Read the model definition and answer for the solid it produces. Units are mm, in the model's axes. Face numbers are marked on the shaded views. A direction names the side the tool comes from. Coordinates: 2 decimals unless noted, no trailing zeros. Order: outer loops, then holes, each group sorted by start corner. A loop starts at its lowest first (then second) coordinate and runs counter-clockwise, first axis right, second up. Notation, with made-up numbers: M 81.5,30 L 136.5,30 A20 ccw 136.5,43 Z; hole C 25,84 d3. An arc over 180 degrees is marked long. Use a Markdown table: item, result. Add a question column.
1) Find section C-C on z = 24.5. Write down the section's boundary in (x, y) (3 decimals).
2) Find the intervals of material crossed by probe 1 along X at (y, z) = (6, 21) (3 decimals); probe 2 along X at (y, z) = (-16.5, 46) (3 decimals); probe 3 along Z at (x, y) = (-22, 2.5) (3 decimals), in increasing order. Write a range as [from, to].
3) Find section A-A on z = 39. Write down the section's boundary in (x, y) (3 decimals), plus the area to 3 significant figures.
4) The mould has two halves that part along X. Classify the marked faces 4, 5 and 6: released by +X, released by -X, zero draft, split by the parting line, or undercut.
5) Find section B-B on x = -10. Write down the section's boundary in (y, z) (3 decimals).
6) Each of these flat-tipped pins is pushed along its axis until it touches: pin 1 Ø3 at (x, y) = (-11.5, 2.5) entering from +Z (3 decimals); pin 2 Ø9.5 at (y, z) = (-18, 46.5) entering from +X (3 decimals); pin 3 Ø12 at (x, z) = (14, 50) entering from -Y (3 decimals); pin 4 Ø9.5 at (y, z) = (-17, 32.5) entering from -X (3 decimals). Where does it stop, or does it pass through?
7) For the marked faces 1, 2 and 3, determine the directions among +Z, -Z, +X, -X, +Y, -Y from which every point of the face is accessible in a straight line to the end or side of a thin tool.
8) Find section D-D on y = 2.5. Write down the section's boundary in (x, z) (3 decimals), plus the area to 3 significant figures.
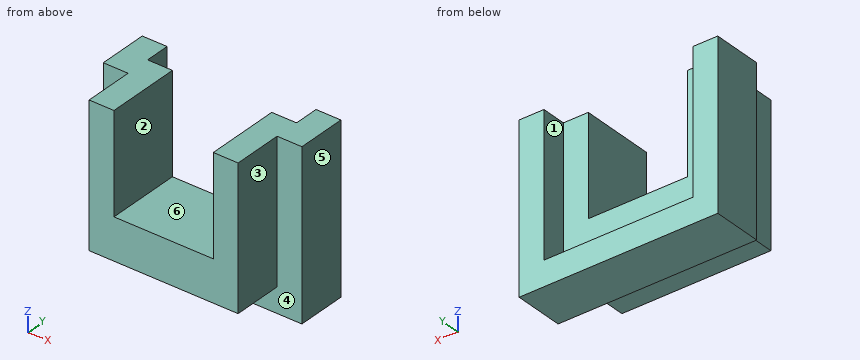
from build123d import *

# Parameters (mm, degrees)
BOSS_EXTRUDE1_DEPTH = 9.525
BOSS_EXTRUDE2_DEPTH = 28.575


with BuildPart() as part:
    # Sketch1 → Boss-Extrude1 (new, symmetric)
    with BuildSketch(Plane(origin=(0, 0, 0), x_dir=(1, 0, 0), z_dir=(0, 1, 0))):
        Polygon((38.1, 0), (-38.1, 0), (-38.1, -63.5), (-28.575, -63.5), (-28.575, -9.525), (28.575, -9.525), (28.575, -63.5), (38.1, -63.5), align=None)
    extrude(amount=BOSS_EXTRUDE1_DEPTH, both=True)

    # Sketch1<3> → Boss-Extrude2 (add)
    with BuildSketch(Plane(origin=(0, 0, 0), x_dir=(1, 0, 0), z_dir=(0, 1, 0))):
        Polygon((-28.575, -9.525), (-28.575, -63.5), (-19.05, -63.5), (-19.05, -25.4), (19.05, -25.4), (19.05, -63.5), (28.575, -63.5), (28.575, -9.525), align=None)
    extrude(amount=-BOSS_EXTRUDE2_DEPTH)


solid = part.part
Check result:
| question | item | result |
|---|---|---|
| 1 | outline | M -38.1,-9.525 L -28.575,-9.525 L -28.575,-28.575 L 28.575,-28.575 L 28.575,-9.525 L 38.1,-9.525 L 38.1,9.525 L 28.575,9.525 L 28.575,0 L -28.575,0 L -28.575,9.525 L -38.1,9.525 Z |
| 2 | probe 1 | x = [-38.1, -28.575], [28.575, 38.1] |
| 2 | probe 2 | x = [-28.575, -19.05], [19.05, 28.575] |
| 2 | probe 3 | z = [0, 9.525] |
| 3 | outline | M -38.1,-9.525 L -28.575,-9.525 L -28.575,-28.575 L -19.05,-28.575 L -19.05,0 L -28.575,0 L -28.575,9.525 L -38.1,9.525 Z; M 19.05,-28.575 L 28.575,-28.575 L 28.575,-9.525 L 38.1,-9.525 L 38.1,9.525 L 28.575,9.525 L 28.575,0 L 19.05,0 Z |
| 3 | area | 907 mm2 |
| 4 | face 4 | zero draft |
| 4 | face 5 | released by +X |
| 4 | face 6 | undercut |
| 5 | outline | M -28.575,9.525 L -9.525,9.525 L -9.525,0 L 9.525,0 L 9.525,9.525 L 0,9.525 L 0,25.4 L -28.575,25.4 Z |
| 6 | pin 1 | stops at z = 9.525 |
| 6 | pin 2 | stops at x = 28.575 |
| 6 | pin 3 | stops at y = -28.575 |
| 6 | pin 4 | stops at x = -28.575 |
| 7 | face 1 | +Z, +Y |
| 7 | face 2 | +Z, +Y, -Y |
| 7 | face 3 | +Z, -Z, +X, -Y |
| 8 | outline | M -38.1,0 L 38.1,0 L 38.1,63.5 L 28.575,63.5 L 28.575,9.525 L -28.575,9.525 L -28.575,63.5 L -38.1,63.5 Z |
| 8 | area | 1,750 mm2 |
